from build123d import *

# Parameters (mm, degrees)
BOSS_EXTRUDE1_DEPTH = 1.5
SKETCH2_W           = 10
SKETCH2_H           = 7.5
BOSS_EXTRUDE2_DEPTH = 10
SKETCH3_R           = 1.6
SKETCH3_R_2         = 0.75
CUT_EXTRUDE1_DEPTH  = 2.5


with BuildPart() as part:
    # Sketch1 → Boss-Extrude1 (new body)
    with BuildSketch(Plane(origin=(0, 0, 0), x_dir=(1, 0, 0), z_dir=(0, 1, 0))):
        with BuildLine():
            Line((-21, 0), (-10, 0))
            Line((-10, 0), (0, 0))
            Line((0, 0), (0, 11))
            Line((0, 11), (-10, 11))
            ThreePointArc((-10, 11), (-17.778174593, 7.778174593), (-21, 0))
        make_face()
        with BuildLine():
            Line((0, 0), (-10, 0))
            Line((-10, 0), (-21, 0))
            ThreePointArc((-21, 0), (-17.778174593, -7.778174593), (-10, -11))
            Line((-10, -11), (0, -11))
            Line((0, -11), (0, 0))
        make_face()
        with BuildLine():
            Line((10, 0), (0, 0))
            Line((0, 0), (0, -11))
            Line((0, -11), (10, -11))
            ThreePointArc((10, -11), (17.778174593, -7.778174593), (21, 0))
            Line((21, 0), (10, 0))
        make_face()
        with BuildLine():
            Line((0, 11), (0, 0))
            Line((0, 0), (10, 0))
            Line((10, 0), (21, 0))
            ThreePointArc((21, 0), (17.778174593, 7.778174593), (10, 11))
            Line((10, 11), (0, 11))
        make_face()
    extrude(amount=BOSS_EXTRUDE1_DEPTH)

    # Sketch2 → Boss-Extrude2 (add)
    with BuildSketch(Plane(origin=(0, 1.5, 0), x_dir=(1, 0, 0), z_dir=(0, 1, 0))):
        with Locations((0, 6.5)):
            Rectangle(SKETCH2_W, SKETCH2_H)
    extrude(amount=BOSS_EXTRUDE2_DEPTH)

    # Sketch3 → Cut-Extrude1 (cut, through all)
    with BuildSketch(Plane(origin=(0, 1.5, 0), x_dir=(1, 0, 0), z_dir=(0, 1, 0))):
        with Locations((0, -9)):
            Circle(SKETCH3_R)
        with Locations((-4, -9.5)):
            Circle(SKETCH3_R_2)
        with Locations((4, -9.5)):
            Circle(SKETCH3_R_2)
    extrude(amount=-CUT_EXTRUDE1_DEPTH, mode=Mode.SUBTRACT)


solid = part.part
Geometry: final body of the model. Coordinates: model frame, mm. A direction names the side the tool comes from. Give positions to 0.01 mm unless a question says otherwise; leave off trailing zeros. Write each loop counter-clockwise with the first axis right and the second up, starting at its lowest first coordinate (ties: lowest second). Pieces come first, ordered by that corner, then holes.
(1) Cut plane D-D, the plane y = 3.25. Return loops of the section in (x, z).
(2) Cut plane B-B, the plane z = 9.5. Return loops of the section in (x, y), then the cut area to 3 significant figures.
(3) First-contact query: P1, Ø1.4, axis at x = -4, z = 9.5, coming from the -Y side; P2, Ø4, axis at x = -8, z = 7, coming from the +Y side; P3, Ø4, axis at y = 8, z = -7, coming from the -X side; P4, Ø3, axis at x = 3.5, y = 3.5, coming from the +Z side. Flat tips, straight axial feed; report the tip coordinate or a pass-through.
(4) Access query for faces 5 (the flat face through (5, 6, -6)), 6 (the cylindrical face through (-0.35, 0.76, 10.56)), 7 (the flat face through (-5, 6, -6)), 8 (the flat face through (0, 6, -2.75)). Directions: +Z, -Z, +X, -X, +Y, -Y. A direction counts if a zero-diameter tool reaches every point of the face in a straight line with its end or side. Return the directions, or none.
(5) Cut plane A-A, the plane x = 0. Return loops of the section in (y, z), then the cut area to 3 significant figures.
(6) Cut plane C-C, the plane x = 6.5. Return loops of the section in (y, z).
(7) Ray query, line 1 (X direction, y = 0.45, z = 9); line 2 (X direction, y = 0.45, z = 9.5); line 3 (Z direction, x = 4, y = 0.75). Return the intervals inside material, ascending.
(8) Mould query, pull axis Z, two halves, no side actions, for faces 1 (the flat face through (0, 6, -10.25)), 2 (the cylindrical face through (-4.55, 0.76, 8.99)), 3 (the flat face through (0, 1, 11)), 4 (the flat face through (0, 1.5, 0)). Classes: released by +Z, released by -Z, zero draft, split by the parting line, or undercut.
Values follow:
1. outline: (-5, -10.25) - (5, -10.25) - (5, -2.75) - (-5, -2.75) - close
2. outline: (-15.55, 0) - (-4.75, 0) - (-4.75, 1.5) - (-15.55, 1.5) - close; (-3.25, 0) - (-1.52, 0) - (-1.52, 1.5) - (-3.25, 1.5) - close; (1.52, 0) - (3.25, 0) - (3.25, 1.5) - (1.52, 1.5) - close; (4.75, 0) - (15.55, 0) - (15.55, 1.5) - (4.75, 1.5) - close
2. area: 37.6 mm2
3. P1: passes through
3. P2: stops at y = 1.5
3. P3: stops at x = -5
3. P4: stops at z = -2.75
4. face 5: +Z, -Z, +X, +Y
4. face 6: +Y, -Y
4. face 7: +Z, -Z, -X, +Y
4. face 8: +Z, +X, -X, +Y
5. outline: (0, -11) - (1.5, -11) - (1.5, -10.25) - (11.5, -10.25) - (11.5, -2.75) - (1.5, -2.75) - (1.5, 7.4) - (0, 7.4) - close; (0, 10.6) - (1.5, 10.6) - (1.5, 11) - (0, 11) - close
5. area: 103 mm2
6. outline: (0, -11) - (1.5, -11) - (1.5, 11) - (0, 11) - close
7. line 1: x = -16.32 to -4.56, -3.44 to -1.6, 1.6 to 3.44, 4.56 to 16.32
7. line 2: x = -15.55 to -4.75, -3.25 to -1.52, 1.52 to 3.25, 4.75 to 15.55
7. line 3: z = -11 to 8.75, 10.25 to 11
8. face 1: released by -Z
8. face 2: undercut
8. face 3: released by +Z
8. face 4: zero draft
